Design review of the part built by this model. Coordinates are the model's own, in mm. A direction names the side the tool comes from. Coordinates: 2 decimals unless noted, no trailing zeros. Write each loop counter-clockwise with the first axis right and the second up, starting at its lowest first coordinate (ties: lowest second). Pieces come first, ordered by that corner, then holes. Notation, with made-up numbers: M -26,-24 L 33,-24 A20 cw 33,-6 Z; hole C 51.25,24.25 d8. An arc over 180 degrees is marked long. One line per question, with ' | ' between items.
from build123d import *

# Parameters (mm, degrees)
SKETCH1_W           = 200
SKETCH1_H           = 100
BOSS_EXTRUDE1_DEPTH = 10
CUT_EXTRUDE1_DEPTH  = 10
BOSS_EXTRUDE2_START = 150
BOSS_EXTRUDE2_DEPTH = 150
BOSS_EXTRUDE3_DEPTH = 80


with BuildPart() as part:
    # Sketch1 → Boss-Extrude1 (new body)
    with BuildSketch(Plane.XY):
        with Locations((100, 50)):
            Rectangle(SKETCH1_W, SKETCH1_H)
    extrude(amount=BOSS_EXTRUDE1_DEPTH)

    # Sketch2 → Cut-Extrude1 (cut)
    with BuildSketch(Plane.XY.offset(10)):
        with BuildLine():
            ThreePointArc((0, 85), (4.393398282, 95.606601718), (15, 100))
            Line((15, 100), (0, 100))
            Line((0, 100), (0, 85))
        make_face()
        with BuildLine():
            Line((200, 100), (185, 100))
            ThreePointArc((185, 100), (195.606601718, 95.606601718), (200, 85))
            Line((200, 85), (200, 100))
        make_face()
        with BuildLine():
            Line((200, 0), (200, 15))
            ThreePointArc((200, 15), (195.606601718, 4.393398282), (185, 0))
            Line((185, 0), (200, 0))
        make_face()
        with BuildLine():
            ThreePointArc((15, 0), (4.393398282, 4.393398282), (0, 15))
            Line((0, 15), (0, 0))
            Line((0, 0), (15, 0))
        make_face()
    extrude(amount=-CUT_EXTRUDE1_DEPTH, mode=Mode.SUBTRACT)

    # Sketch3 → Boss-Extrude2 (add)
    with BuildSketch(Plane.XY.offset(10).offset(BOSS_EXTRUDE2_START)):
        with BuildLine():
            Line((100, 100), (185, 100))
            ThreePointArc((185, 100), (195.606601718, 95.606601718), (200, 85))
            Line((200, 85), (200, 15))
            ThreePointArc((200, 15), (195.606601718, 4.393398282), (185, 0))
            Line((185, 0), (15, 0))
            ThreePointArc((15, 0), (4.393398282, 4.393398282), (0, 15))
            Line((0, 15), (0, 85))
            ThreePointArc((0, 85), (4.393398282, 95.606601718), (15, 100))
            Line((15, 100), (100, 100))
        make_face()
        with BuildLine():
            Line((30, 95), (170, 95))
            ThreePointArc((170, 95), (187.67766953, 87.67766953), (195, 70))
            Line((195, 70), (195, 30))
            ThreePointArc((195, 30), (187.67766953, 12.32233047), (170, 5))
            Line((170, 5), (30, 5))
            ThreePointArc((30, 5), (12.32233047, 12.32233047), (5, 30))
            Line((5, 30), (5, 70))
            ThreePointArc((5, 70), (12.32233047, 87.67766953), (30, 95))
        make_face(mode=Mode.SUBTRACT)
    extrude(amount=-BOSS_EXTRUDE2_DEPTH)

    # Sketch4 → Boss-Extrude3 (add)
    with BuildSketch(Plane.XY.offset(10)):
        Polygon((66, 60.5), (56, 60.5), (56, 39.5), (66, 39.5), (66, 49.5), (65, 49.5), (65, 50), (65, 50.5), (66, 50.5), align=None)
        Polygon((144, 39.5), (134, 39.5), (134, 49.5), (135, 49.5), (135, 50), (135, 50.5), (134, 50.5), (134, 60.5), (144, 60.5), align=None)
    extrude(amount=BOSS_EXTRUDE3_DEPTH)


solid = part.part
1. Take a section at C-C (y = 44). Write out the cut boundary in (x, z), then the cut area to 3 significant figures.
Answer sheet:
outline: M 0,0 L 200,0 L 200,160 L 195,160 L 195,10 L 144,10 L 144,90 L 134,90 L 134,10 L 66,10 L 66,90 L 56,90 L 56,10 L 5,10 L 5,160 L 0,160 Z | area: 5,100 mm^2
2. Take a section at D-D (x = 141.5). Write out the cut boundary in (y, z).
Answer sheet:
outline: M 0,0 L 100,0 L 100,160 L 95,160 L 95,10 L 60.5,10 L 60.5,90 L 39.5,90 L 39.5,10 L 5,10 L 5,160 L 0,160 Z
3. Insertion check: pin 1 Ø2 at (x, y) = (112.5, 17.5) entering from +Z; pin 2 Ø10 at (x, y) = (92, 78) entering from -Z; pin 3 Ø5 at (x, y) = (63, 48.5) entering from +Z. Each pin has a flat end and moves straight along its axis. Give the tip position at first contact, or say it passes through.
Answer sheet:
pin 1: z = 10 | pin 2: z = 0 | pin 3: z = 90
4. Draft analysis for pull direction Y (two halves, no side actions). For faces 3 (the face through (101, 0, 81)), 4 (the face through (0, 50, 81)), 5 (the face through (139, 60.5, 49)), 6 (the face through (101, 5, 86)), state which applies: pulls with the +Y half, pulls with the -Y half, needs draft (parallel to the pull), parting line crosses it, or undercut.
Answer sheet:
face 3: pulls with the -Y half | face 4: needs draft | face 5: undercut | face 6: undercut
5. Tool access review of faces 1 (the face through (200, 50, 81)), 2 (the face through (61, 39.5, 49)): name each direction out of +Z, -Z, +X, -X, +Y, -Y from which nothing blocks a thin tool from reaching the whole face with its end or side.
Answer sheet:
face 1: +Z, -Z, +X, +Y, -Y | face 2: +Z
6. Take a section at A-A (z = 45). Count the separate pieces of the cut face and the enclosed holes in it, then the cut area to 3 significant figures.
Answer sheet:
separate pieces: 3 | enclosed holes: 1 | area: 3,660 mm^2
7. To check wall thickness, follow line 1 along X through (y, z) = (49, 51.5); line 2 along Y through (x, z) = (138.5, 124.5); line 3 along X through (y, z) = (33.5, 57). State the ranges of each line that lie inside material, in increasing order. Write a range as [from, to].
Answer sheet:
line 1: [0, 5], [56, 66], [134, 144], [195, 200] | line 2: [0, 5], [95, 100] | line 3: [0, 5], [195, 200]
8. Take a section at B-B (z = 109.5). Write out the cut boundary in (x, y), then the cut area to 3 significant figures.
Answer sheet:
outline: M 0,15 A15 ccw 15,0 L 185,0 A15 ccw 200,15 L 200,85 A15 ccw 185,100 L 15,100 A15 ccw 0,85 Z; hole M 5,30 A25 ccw 30,5 L 170,5 A25 ccw 195,30 L 195,70 A25 ccw 170,95 L 30,95 A25 ccw 5,70 Z | area: 3,240 mm^2
